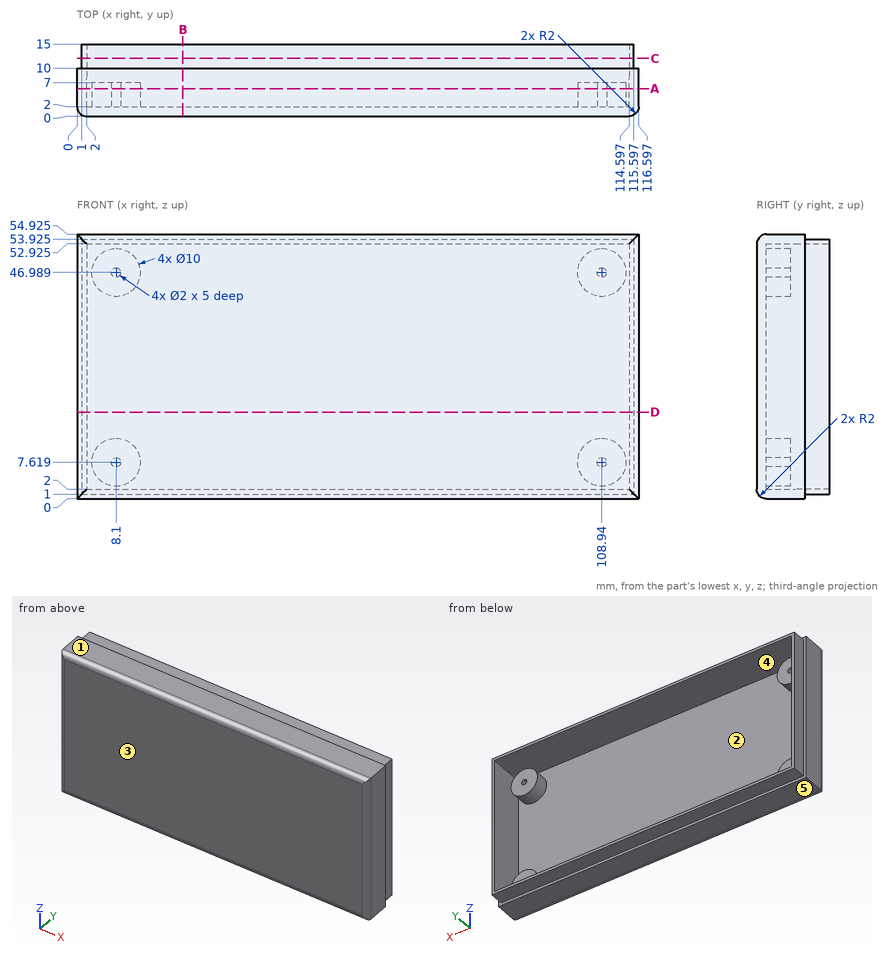
Design review of the part shown in the three views and the two pictorial views. Dimensions are in mm from the part's minimum x, y and z. A direction names the side the tool comes from. Coordinates: 2 decimals unless noted, no trailing zeros. Loops run counter-clockwise (first coordinate to the right, second up) from the corner with the lowest first, then second, coordinate; pieces in that order, holes last.
Q1. We need section C-C on y = 12. State the section outline as (x, z) points (1 decimal).
Reported:
outline: (1, 1) - (115.6, 1) - (115.6, 53.9) - (1, 53.9) - close; hole (2, 2) - (114.6, 2) - (114.6, 52.9) - (2, 52.9) - close
Q2. We need section D-D on z = 18. State the section outline as (x, y) points.
Reported:
outline: (0, 2) arc R2 ccw to (2, 0) - (114.6, 0) arc R2 ccw to (116.6, 2) - (116.6, 10) - (115.6, 10) - (115.6, 15) - (114.6, 15) - (114.6, 2) - (2, 2) - (2, 15) - (1, 15) - (1, 10) - (0, 10) - close
Q3. For pin 1 (10 mm diameter, centred on x = 56, z = 43, fed in from +Y); pin 2 (1.6 mm diameter, centred on x = 109, z = 8, fed in from +Y); pin 3 (2.5 mm diameter, centred on x = 54, y = 12.5, fed in from +Z) (1 decimal), all flat-tipped, find the tip position at first contact; note any pin that passes through.
Reported:
pin 1: stops at y = 2
pin 2: stops at y = 7
pin 3: stops at z = 53.9
Q4. We need section A-A on y = 5.75. State how many separate pieces and enclosed holes the cut face has.
Reported:
separate pieces: 5
enclosed holes: 5
Q5. Tool access review of the marked faces 4 and 5: name each direction out of +Z, -Z, +X, -X, +Y, -Y from which nothing blocks a thin tool from reaching the whole face with its end or side.
Reported:
face 4: +Y
face 5: -Z, +X, -X, +Y, -Y
Q6. We need section B-B on x = 22. State the section outline as (y, z) points (1 decimal).
Reported:
outline: (0, 2) arc R2 ccw to (2, 0) - (10, 0) - (10, 1) - (15, 1) - (15, 2) - (2, 2) - (2, 52.9) - (15, 52.9) - (15, 53.9) - (10, 53.9) - (10, 54.9) - (2, 54.9) arc R2 ccw to (0, 52.9) - close
Q7. To check wall thickness, follow line 1 (Z direction, x = 62.5, y = 5) (1 decimal); line 2 (Z direction, x = 65.5, y = 12) (1 decimal); line 3 (X direction, y = 5.5, z = 5). State the ranges of each line that lie inside material, in increasing order.
Reported:
line 1: z = 0 to 2, 52.9 to 54.9
line 2: z = 1 to 2, 52.9 to 53.9
line 3: x = 0 to 2, 3.84 to 12.36, 104.68 to 113.2, 114.6 to 116.6
Q8. The part is to be moulded in two halves that separate along Z. For the marked faces 1, 2 and 3, say which applies: +Z half, -Z half, draft (parallel to the pull), parting line (faces both ways), or undercut.
Reported:
face 1: +Z half
face 2: undercut
face 3: draft
